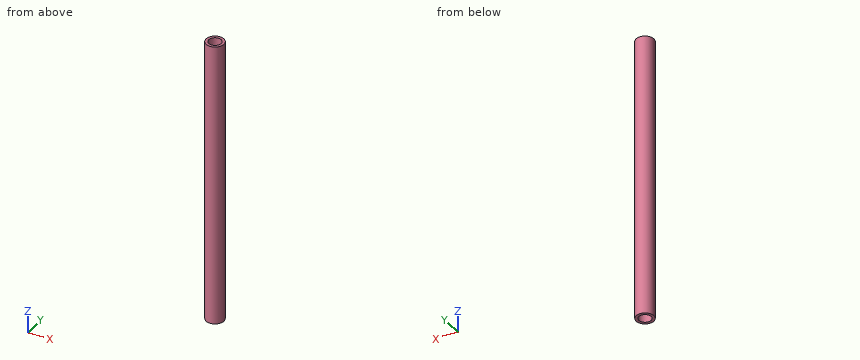
Autodesk Inventor part; units mm, degrees
ref_plane "YZ Plane" through (0, 0, 0) normal (1, 0, 0) x (0, 1, 0)
ref_plane "XZ Plane" through (0, 0, 0) normal (0, 1, 0) x (-1, 0, 0)
ref_plane "XY Plane" through (0, 0, 0) normal (0, 0, 1) x (1, 0, 0)
sketch "Sketch1" plane through (0, 0, 0) normal (0, 0, 1) x (1, 0, 0)
  circle A0 centre (0, 0) radius 2.3813
  dimension "d0" = 4.7625
extrude "Extrusion1" add sketch "Sketch1" along normal blind 76.2
sketch "Sketch2" plane through (0, 0, 76.2) normal (0, 0, 1) x (1, 0, 0)
  circle A0 centre (0, 0) radius 2.3813
  circle A1 centre (0, 0) radius 1.1303
  dimension "d3" = 2.2606
hole "Hole1" at (0, 0, 76.2) direction (0, 0, -1) diameter 3.302 depth 12.2936 tip angle 118
sketch "Sketch3" plane through (0, 0, 0) normal (0, 0, -1) x (-1, 0, 0)
  circle A0 centre (0, 0) radius 2.3813
hole "Hole2" at (0, 0, 0) direction (0, 0, 1) diameter 3.302 depth 12.2936 tip angle 118
properties part number "Steel Rod"
Source: CAD feature listing. Evaluate the final solid. Frame: model axes, mm. Round coordinates to 2 decimals unless told otherwise and drop trailing zeros. Loops run counter-clockwise (first coordinate to the right, second up) from the corner with the lowest first, then second, coordinate; pieces in that order, holes last.
1. Section query A-A on z = 40.5. Output: boundary loops of the cut face in (x, y).
2. Ray query, L1, parallel to X at y = 0.2, z = 64; L2, parallel to Y at x = 0, z = 9.5; L3, parallel to Y at x = 0.15, z = 36. Return the intervals inside material, ascending.
3. Contact query for a flat-ended pin moving along its axis: pin 1 (1.5 mm diameter, centred on x = -1, z = 40.5, fed in from -Y). Output: stop coordinate, or through.
Answers below:
1. outline: circle Ø4.76 at (0, 0)
2. L1: x = -2.37 to -1.64, 1.64 to 2.37
2. L2: y = -2.38 to -1.65, 1.65 to 2.38
2. L3: y = -2.38 to 2.38
3. pin 1: stops at y = -2.37
